Check sheet for the drawn part. Datum: minimum x, y, z corner. Units: mm. Give positions to 0.01 mm unless a question says otherwise; leave off trailing zeros. Order: outer loops, then holes, each group sorted by start corner. A loop starts at its lowest first (then second) coordinate and runs counter-clockwise, first axis right, second up. Notation, with made-up numbers: (-33.75, 30.25) -> (-29.75, 30.25) arc R26 ccw to (-29.75, 67.25) -> close; hole circle Ø10 at (-18.5, 14). An arc over 180 degrees is marked (long way). Return JSON: item names as keys, results as strings. Group by question number.
(1) Depth check by flat-ended pin: pin 1 Ø12 at (x, y) = (18, 54.5) entering from +Z; pin 2 Ø1.5 at (x, z) = (16.5, 3) entering from -Y (1 decimal); pin 3 Ø2 at (x, z) = (15, 3) entering from -Y (1 decimal). Enter the tip coordinate at first touch or a pass-through.
(2) Cross-section at C-C on x = 19. Enter the section's corners in (y, z) (1 decimal).
(3) Thickness scan on line 1 along X through (y, z) = (118.5, 6.25); line 2 along Z through (x, y) = (16.5, 73); line 3 along Y through (x, z) = (23.5, 8.75) (1 decimal). Record the ranges inside material, lowest first.
(4) Cross-section at B-B on z = 2.75. Enter the section's corners in (x, y), then the cut area to 3 significant figures.
(5) Release check for a two-part mould opening along Y. For the marked faces 1, 2 and 3 record: pulls with the +Y half, pulls with the -Y half, needs draft (parallel to the pull), parting line crosses it, or undercut.
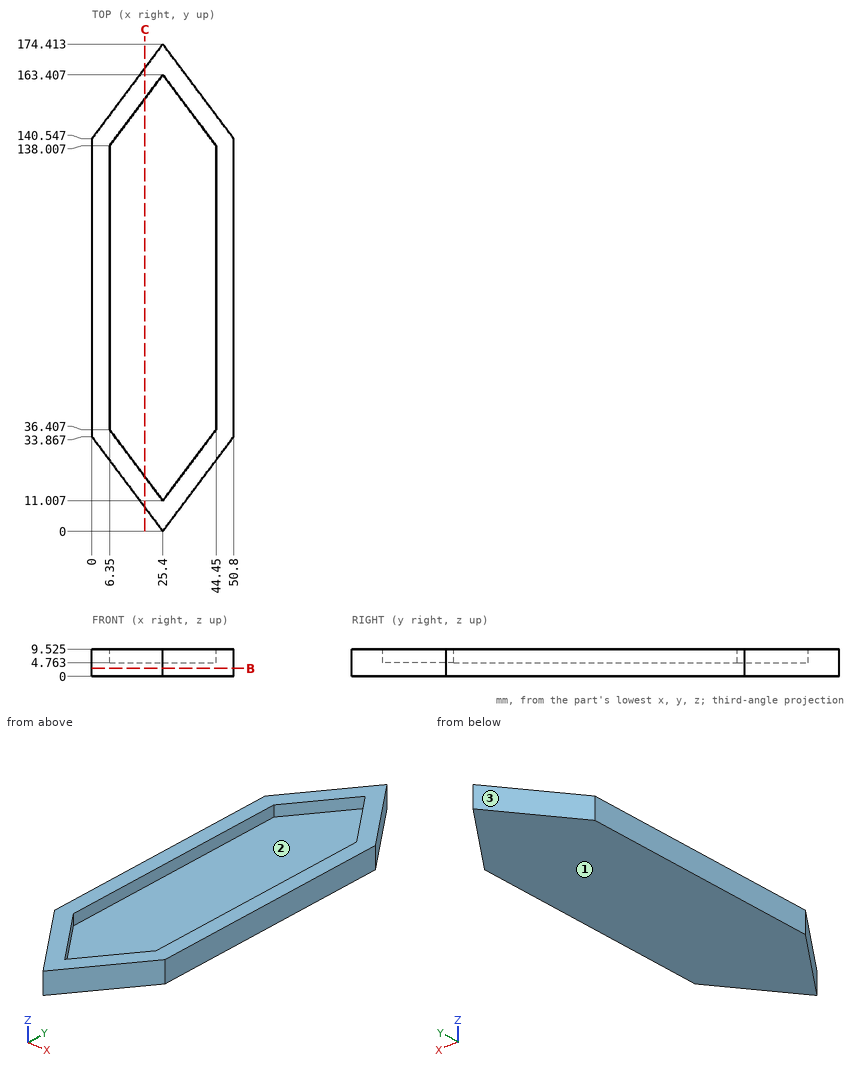
Verdict:
{
 "1": {"pin 1": "z = 4.76", "pin 2": "y = 10.9", "pin 3": "y = 12.5"},
 "2": {"outline": "(8.5, 0) -> (165.9, 0) -> (165.9, 9.5) -> (154.9, 9.5) -> (154.9, 4.8) -> (19.5, 4.8) -> (19.5, 9.5) -> (8.5, 9.5) -> close"},
 "3": {"line 1": "0 to 6.35, 44.45 to 50.8", "line 2": "0 to 4.76", "line 3": "2.5 to 13.5, 160.9 to 171.9"},
 "4": {"outline": "(0, 33.87) -> (25.4, 0) -> (50.8, 33.87) -> (50.8, 140.55) -> (25.4, 174.41) -> (0, 140.55) -> close", "area": "7,140 mm²"},
 "5": {"face 1": "needs draft", "face 2": "undercut", "face 3": "pulls with the +Y half"}
}
